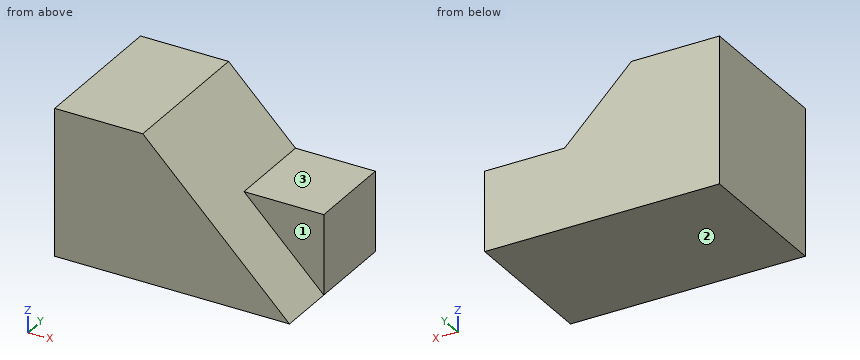
from build123d import *

# Parameters (mm, degrees)
F0_W     = 50.8
F0_H     = 31.75
F1_DEPTH = 31.75
F3_DEPTH = 12.7
F5_DEPTH = 25.4
F7_DEPTH = 25.4


with BuildPart() as f1:
    # F0 (on Front) → F1 (new body)
    with BuildSketch(Plane.XZ):
        with Locations((25.4, 15.875)):
            Rectangle(F0_W, F0_H)
    extrude(amount=F1_DEPTH)

    # F2 (on face) → F3 (cut)
    with BuildSketch(Plane.XZ.offset(31.75)):
        Polygon((50.8, 31.75), (19.05, 31.75), (50.8, 0), align=None)
    extrude(amount=-F3_DEPTH, mode=Mode.SUBTRACT)

    # F4 (on face) → F5 (cut)
    with BuildSketch(Plane(origin=(0, 0, 0), x_dir=(-1, 0, 0), z_dir=(0, 1, 0))):
        Polygon((-38.1, 17.2671154141), (-25.4, 31.75), (-50.8, 31.75), (-50.8, 17.2671154141), align=None)
    extrude(amount=-F5_DEPTH, mode=Mode.SUBTRACT)

    # F6 (on face) → F7 (cut)
    with BuildSketch(Plane.XZ.offset(19.05)):
        Polygon((33.5328845859, 17.2671154141), (38.1, 17.2671154141), (25.4, 31.75), (19.05, 31.75), align=None)
    extrude(amount=-F7_DEPTH, mode=Mode.SUBTRACT)


solid = f1.part
The model under review builds one solid part; all positions refer to its coordinate system, in mm. Face numbers are marked on the shaded views. A direction names the side the tool comes from. Round coordinates to 2 decimals unless told otherwise and drop trailing zeros. Write each loop counter-clockwise with the first axis right and the second up, starting at its lowest first coordinate (ties: lowest second). Pieces come first, ordered by that corner, then holes. Notation, with made-up numbers: M 34.5,-8.5 L 73.5,-8.5 A16 ccw 73.5,5.5 Z; hole C 39.5,32 d2. An arc over 180 degrees is marked long. Use a Markdown table: item, result. Add a question column.
Q1. To check wall thickness, follow line 1 (X direction, y = -22, z = 9); line 2 (Z direction, x = 31.5, y = -26.5); line 3 (X direction, y = -21, z = 23). State the ranges of each line that lie inside material, in increasing order.
Q2. We need section D-D, the plane x = 22. State the section outline as (y, z) points.
Q3. Machinability: for the marked faces 1, 2 and 3, which of the approach directions +Z, -Z, +X, -X, +Y, -Y give a long, thin tool a straight path to every point of the face, cutting with its end or side? Answer none if there is none.
Q4. Insertion check: pin 1 (1 mm diameter, centred on y = -16.5, z = 24, fed in from +X); pin 2 (3 mm diameter, centred on x = 31, y = -13, fed in from +Z); pin 3 (3 mm diameter, centred on x = 27, y = -11.5, fed in from +Z). Each pin has a flat end and moves straight along its axis. Give the tip position at first contact, or say it passes through.
Q5. We need section B-B, the plane x = 38. State the section outline as (y, z) points.
Q6. We need section A-A, the plane z = 5.5. State the section outline as (x, y) points.
Q7. We need section C-C, the plane y = -26.5. State the section outline as (x, z) points, plus the area to 3 significant figures.
Findings below:
| question | item | result |
|---|---|---|
| 1 | line 1 | x = 0 to 41.8 |
| 1 | line 2 | z = 0 to 19.3 |
| 1 | line 3 | x = 0 to 27.8 |
| 2 | outline | M -31.75,0 L 0,0 L 0,28.8 L -31.75,28.8 Z |
| 3 | face 1 | +Z, +X, -Y |
| 3 | face 2 | -Z, +X, -X, +Y, -Y |
| 3 | face 3 | +Z, +X, +Y, -Y |
| 4 | pin 1 | stops at x = 27.3 |
| 4 | pin 2 | stops at z = 21.3 |
| 4 | pin 3 | stops at z = 25.3 |
| 5 | outline | M -31.75,0 L 0,0 L 0,17.27 L -19.05,17.27 L -19.05,12.8 L -31.75,12.8 Z |
| 6 | outline | M 0,-31.75 L 45.3,-31.75 L 45.3,-19.05 L 50.8,-19.05 L 50.8,0 L 0,0 Z |
| 7 | outline | M 0,0 L 50.8,0 L 19.05,31.75 L 0,31.75 Z |
| 7 | area | 1,110 mm² |
